Check sheet for the modelled part. Datum: model origin and axes. Units: mm. A direction names the side the tool comes from. Coordinates: 2 decimals unless noted, no trailing zeros. Loops run counter-clockwise (first coordinate to the right, second up) from the corner with the lowest first, then second, coordinate; pieces in that order, holes last. Notation, with made-up numbers: (25, 6.25) - (55, 6.25) arc R9 cw to (55, 13.25) - close; hole circle Ø8 at (-2.5, 71.25). An arc over 180 degrees is marked (long way). Use a Markdown table: item, result. Add a question column.
1) Draft check along Y on faces 1 (the flat face through (-6, -1.172, 11)), 2 (the cylindrical face through (-3.015, 5.754, 0.986)), 3 (the cylindrical face through (-16.616, 0.349, 15.301)), 4 (the cylindrical face through (-4.366, 2.113, 3.301)). Enter one of: pulls with the +Y half, pulls with the -Y half, needs draft (parallel to the pull), parting line crosses it, or undercut.
2) Sectioned sample at C-C, the plane x = -9. Enter the section's corners in (y, z), then the cut area to 3 significant figures.
3) Sectioned sample at A-A, the plane y = 1.5. Enter the section's corners in (x, z), then the cut area to 3 significant figures.
4) Sectioned sample at B-B, the plane z = 11.75. Enter the section's corners in (x, y).
5) Go/stop test with flat-tipped pins: P1, Ø2.5, axis at x = -12.5, y = 1, coming from the -Z side; P2, Ø5, axis at x = -4.4, y = 6.33, coming from the +Z side. Record where each tip stops, or that it passes through.
6) Thickness scan on line 1 (X direction, y = -0.25, z = 14); line 2 (Y direction, x = -5.25, z = 13.5); line 3 (Z direction, x = -5.25, y = 3.5). Record the ranges inside material, lowest first.
7) Tool access check on faces 5 (the flat face through (-6, 1.828, 12)), 6 (the flat face through (-6.901, 1.5, 5.3)), 7 (the cylindrical face through (-2.202, 0.349, 17.715)). Record the directions out of +Z, -Z, +X, -X, +Y, -Y that give a thin tool (end or side, any length) a straight path to the whole face; none if there is none.
from build123d import *

# Parameters (mm, degrees)
SKETCH1_W           = 5
SKETCH1_H           = 10
SKETCH1_R           = 1.5
BOSS_EXTRUDE1_DEPTH = 3
SKETCH2_W           = 5
SKETCH2_H           = 3
BOSS_EXTRUDE2_DEPTH = 15
SKETCH3_W           = 3
SKETCH3_H           = 3
BOSS_EXTRUDE3_DEPTH = 10
FILLET1_R           = 1
FILLET2_R           = 1
FILLET3_R           = 1
FILLET4_R           = 1
FILLET5_R           = 1
FILLET6_R           = 1
FILLET7_R           = 1


with BuildPart() as part:
    # Sketch1 → Boss-Extrude1 (new body)
    with BuildSketch(Plane.XY):
        with Locations((-4.401041667, 3.828125)):
            Rectangle(SKETCH1_W, SKETCH1_H)
        with Locations((-4.401041667, 6.328125)):
            Circle(SKETCH1_R, mode=Mode.SUBTRACT)
    extrude(amount=BOSS_EXTRUDE1_DEPTH)

    # Sketch2 → Boss-Extrude2 (add)
    with BuildSketch(Plane.XY.offset(3)):
        with Locations((-4.401041667, 0.328125)):
            Rectangle(SKETCH2_W, SKETCH2_H)
    extrude(amount=BOSS_EXTRUDE2_DEPTH)

    # Sketch3 → Boss-Extrude3 (add)
    with BuildSketch(Plane.ZY.offset(6.901041667)):
        with Locations((16.5, 0.328125)):
            Rectangle(SKETCH3_W, SKETCH3_H)
    extrude(amount=BOSS_EXTRUDE3_DEPTH)

    # Fillet1
    fillet1_edges = [part.edges().sort_by_distance(p)[0] for p in [
        (-6.901041667, 0.328125, 15),
    ]]
    fillet(fillet1_edges, radius=FILLET1_R)

    # Fillet2
    fillet2_edges = [part.edges().sort_by_distance(p)[0] for p in [
        (-1.901041667, 0.328125, 18),
    ]]
    fillet(fillet2_edges, radius=FILLET2_R)

    # Fillet3
    fillet3_edges = [part.edges().sort_by_distance(p)[0] for p in [
        (-16.901041667, 0.328125, 15),
    ]]
    fillet(fillet3_edges, radius=FILLET3_R)

    # Fillet4
    fillet4_edges = [part.edges().sort_by_distance(p)[0] for p in [
        (-16.901041667, 0.328125, 18),
    ]]
    fillet(fillet4_edges, radius=FILLET4_R)

    # Fillet5
    fillet5_edges = [part.edges().sort_by_distance(p)[0] for p in [
        (-5.901041667, 6.328125, 3),
    ]]
    fillet(fillet5_edges, radius=FILLET5_R - 0.0001)  # a hair under: the kernel refuses the full size

    # Fillet6
    fillet6_edges = [part.edges().sort_by_distance(p)[0] for p in [
        (-4.401041667, -1.171875, 0),
    ]]
    fillet(fillet6_edges, radius=FILLET6_R)

    # Fillet7
    fillet7_edges = [part.edges().sort_by_distance(p)[0] for p in [
        (-4.401041667, 1.828125, 3),
    ]]
    fillet(fillet7_edges, radius=FILLET7_R)


solid = part.part
Solved:
| question | item | result |
|---|---|---|
| 1 | face 1 | pulls with the -Y half |
| 1 | face 2 | undercut |
| 1 | face 3 | needs draft |
| 1 | face 4 | pulls with the +Y half |
| 2 | outline | (-1.17, 15) - (1.83, 15) - (1.83, 18) - (-1.17, 18) - close |
| 2 | area | 9.00 mm2 |
| 3 | outline | (-16.9, 16) arc R1 ccw to (-15.9, 15) - (-7.9, 15) arc R1 cw to (-6.9, 14) - (-6.9, 0) - (-1.9, 0) - (-1.9, 17) arc R1 ccw to (-2.9, 18) - (-15.9, 18) arc R1 ccw to (-16.9, 17) - close |
| 3 | area | 120 mm2 |
| 4 | outline | (-6.9, -1.17) - (-1.9, -1.17) - (-1.9, 1.83) - (-6.9, 1.83) - close |
| 5 | P1 | stops at z = 15 |
| 5 | P2 | stops at z = 3 |
| 6 | line 1 | x = -6.9 to -1.9 |
| 6 | line 2 | y = -1.17 to 1.83 |
| 6 | line 3 | z = 0 to 3 |
| 7 | face 5 | +Z, +X, -X, +Y |
| 7 | face 6 | -Z, -X, +Y, -Y |
| 7 | face 7 | +Z, +X, +Y, -Y |
